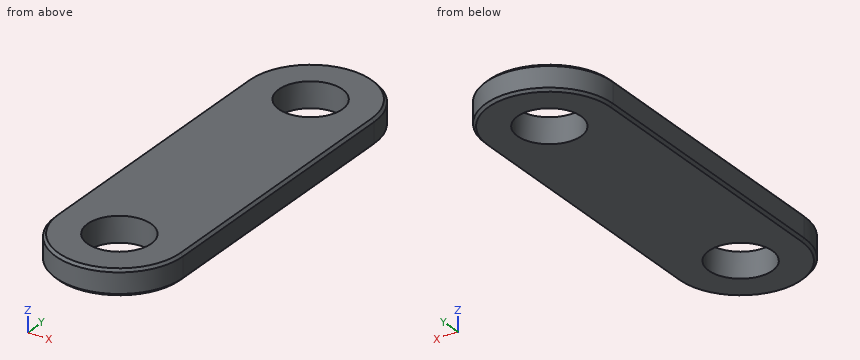
```python
from build123d import *

# Parameters (mm, degrees)
BOSS_EXTRUDE1_DEPTH = 20
SKETCH1_3_R         = 25
CUT_EXTRUDE1_DEPTH  = 149
CHAMFER1_SIZE       = 2


with BuildPart() as part:
    # Sketch1 → Boss-Extrude1 (new body)
    with BuildSketch(Plane.XY):
        with BuildLine():
            Line((-50, 111.475422903), (-50, -113.524577097))
            ThreePointArc((-50, -113.524577097), (0, -163.524577097), (50, -113.524577097))
            Line((50, -113.524577097), (50, 111.475422903))
            ThreePointArc((50, 111.475422903), (0, 161.475422903), (-50, 111.475422903))
        make_face()
    extrude(amount=BOSS_EXTRUDE1_DEPTH)

    # Sketch1<3> → Cut-Extrude1 (cut)
    with BuildSketch(Plane.XY):
        with Locations((0, 111.475422903)):
            Circle(SKETCH1_3_R)
        with Locations((0, -113.524577097)):
            Circle(SKETCH1_3_R)
    extrude(amount=CUT_EXTRUDE1_DEPTH, mode=Mode.SUBTRACT)

    # Chamfer1
    chamfer1_edges = [part.edges().sort_by_distance(p)[0] for p in [
        (0, -163.524577097, 20),
        (50, -1.024577097, 20),
        (0, 161.475422903, 20),
        (50, -1.024577097, 0),
        (0, -163.524577097, 0),
        (-50, -1.024577097, 0),
        (0, 161.475422903, 0),
        (-50, -1.024577097, 20),
    ]]
    chamfer(chamfer1_edges, length=CHAMFER1_SIZE)


solid = part.part
```
Here's how the part is built. I have some questions about the finished solid (model axes, mm). Give positions to 0.01 mm unless a question says otherwise; leave off trailing zeros. Loops run counter-clockwise (first coordinate to the right, second up) from the corner with the lowest first, then second, coordinate; pieces in that order, holes last. Notation, with made-up numbers: (9, -30.5) -> (27, -30.5) arc R17 cw to (27, -19.5) -> close; hole circle Ø3 at (11.25, 67.5). An arc over 180 degrees is marked (long way). Use one line per item in the form item = value. Start each with the question number.
1) For P1, Ø5, axis at x = -3.5, z = 12.5, coming from the -Y side; P2, Ø12, axis at x = 33, z = 7.5, coming from the +Y side; P3, Ø10, axis at x = 35.5, z = 13.5, coming from the +Y side, each with a flat end and sliding along its axis, tell me the tip position at first contact or that it passes through.
2) Please list where these lines run through material, in increasing order: line 1 along Y through (x, z) = (0, 4); line 2 along Y through (x, z) = (2, 4.25); line 3 along X through (y, z) = (112.5, 10.5).
3) Imagine slicing it at C-C (y = -95). Please give me the cut outline in (x, z), then the cut area to 3 significant figures.
4) Imagine slicing it at B-B (z = 11). Please give me the cut outline in (x, y).
5) Imagine slicing it at A-A (x = 0). Please give me the cut outline in (y, z).
Check values:
q1.P1 = -163.51
q1.P2 = 153.56
q1.P3 = 151.1
q2.line_1 = -163.52 to -138.52, -88.52 to 86.48, 136.48 to 161.48
q2.line_2 = -163.48 to -138.44, -88.6 to 86.56, 136.4 to 161.44
q2.line_3 = -49.99 to -24.98, 24.98 to 49.99
q3.outline = (-50, 2) -> (-48, 0) -> (-16.79, 0) -> (-16.79, 20) -> (-48, 20) -> (-50, 18) -> close; (16.79, 0) -> (48, 0) -> (50, 2) -> (50, 18) -> (48, 20) -> (16.79, 20) -> close
q3.area = 1,320 mm^2
q4.outline = (-50, -113.52) arc R50 ccw to (50, -113.52) -> (50, 111.48) arc R50 ccw to (-50, 111.48) -> close; hole circle Ø50 at (0, -113.52); hole circle Ø50 at (0, 111.48)
q5.outline = (-163.52, 2) -> (-161.52, 0) -> (-138.52, 0) -> (-138.52, 20) -> (-161.52, 20) -> (-163.52, 18) -> close; (-88.52, 0) -> (86.48, 0) -> (86.48, 20) -> (-88.52, 20) -> close; (136.48, 0) -> (159.48, 0) -> (161.48, 2) -> (161.48, 18) -> (159.48, 20) -> (136.48, 20) -> close
